Verification items for the finished model (mm, model axes). Round coordinates to 2 decimals unless told otherwise and drop trailing zeros. Loops run counter-clockwise (first coordinate to the right, second up) from the corner with the lowest first, then second, coordinate; pieces in that order, holes last. Notation, with made-up numbers: (57, 40) -> (85, 40) arc R21 ccw to (85, 53) -> close; hole circle Ø7 at (89, 54). An arc over 180 degrees is marked (long way). Write item = value, one per line. Start each with the question number.
```python
from build123d import *

# Parameters (mm, degrees)
SKETCH_1_R      = 1.2
SKETCH_1_R_2    = 1.35
SKETCH_1_R_3    = 1.32
EXTRUDE_1_DEPTH = 3


with BuildPart() as part:
    # 草图1 → 凸台-拉伸1 (new body)
    with BuildSketch(Plane(origin=(0, 0, 0), x_dir=(-1, 0, 0), z_dir=(0, 0, -1))):
        with BuildLine():
            Line((91.218663814, 7.514094575), (60.426417561, 7.514094575))
            ThreePointArc((60.426417561, 7.514094575), (55.954281606, 9.514094575), (51.482145651, 7.514094575))
            Line((51.482145651, 7.514094575), (-24.019834979, 7.514094575))
            ThreePointArc((-24.019834979, 7.514094575), (-28.019834979, 3.514094575), (-24.019834979, -0.485905425))
            Line((-24.019834979, -0.485905425), (51.482145651, -0.485905425))
            ThreePointArc((51.482145651, -0.485905425), (55.954281606, -2.485905425), (60.426417561, -0.485905425))
            Line((60.426417561, -0.485905425), (91.218663814, -0.485905425))
            ThreePointArc((91.218663814, -0.485905425), (95.218663814, 3.514094575), (91.218663814, 7.514094575))
        make_face()
        with Locations(Location((-24.020396654, 3.514094575, 0), (0, 0, 180))):
            Circle(SKETCH_1_R, mode=Mode.SUBTRACT)
        with Locations(Location((55.954281606, 3.514094575, 0), (0, 0, 180))):
            Circle(SKETCH_1_R_2, mode=Mode.SUBTRACT)
        with Locations(Location((91.218663814, 3.514094575, 0), (0, 0, 180))):
            Circle(SKETCH_1_R_3, mode=Mode.SUBTRACT)
    extrude(amount=-EXTRUDE_1_DEPTH)


solid = part.part
```
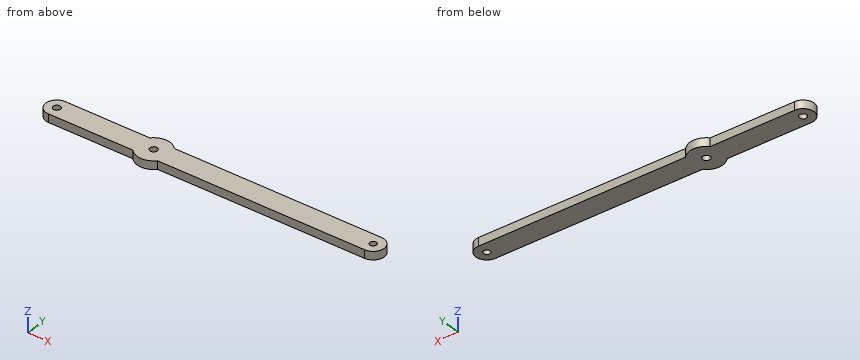
(1) Depth check by flat-ended pin: pin 1 Ø3 at (x, y) = (24.02, 3.51) entering from -Z. Enter the tip coordinate at first touch or a pass-through.
(2) Scan lines: line 1 (X direction, y = 4.25, z = 2.1); line 2 (X direction, y = 4, z = 1.55); line 3 (Y direction, x = -69.5, z = 1.6). Record each from-to range of solid material in increasing order. Write a range as [from, to].
(3) Section check B-B on x = -82.5. Enter the section's corners in (y, z).
(4) Section check A-A on z = 0.85. Enter the section's corners in (x, y), then the cut area to 3 significant figures.
Computed values:
q1.pin_1 = 0
q2.line_1 = [-95.15, -92.31], [-90.12, -57.09], [-54.82, 23.07], [24.97, 27.95]
q2.line_2 = [-95.19, -92.45], [-89.99, -57.21], [-54.69, 22.92], [25.12, 27.99]
q2.line_3 = [-0.49, 7.51]
q3.outline = (-0.49, 0) -> (7.51, 0) -> (7.51, 3) -> (-0.49, 3) -> close
q4.outline = (-91.22, -0.49) -> (-60.43, -0.49) arc R6 ccw to (-51.48, -0.49) -> (24.02, -0.49) arc R4 ccw to (24.02, 7.51) -> (-51.48, 7.51) arc R6 ccw to (-60.43, 7.51) -> (-91.22, 7.51) arc R4 ccw to start; hole circle Ø2.64 at (-91.22, 3.51); hole circle Ø2.7 at (-55.95, 3.51); hole circle Ø2.4 at (24.02, 3.51)
q4.area = 981 mm²
